```python
from build123d import *

# Parameters (mm, degrees)
EXTRUDE_1_DEPTH     = 165
SKETCH_2_W          = 10
SKETCH_2_H          = 150
CUT_EXTRUDE_1_DEPTH = 185.106287236
SKETCH_3_W          = 8
SKETCH_3_H          = 155
EXTRUDE_2_DEPTH     = 10
SKETCH_4_R          = 2.5
CUT_EXTRUDE_2_DEPTH = 180.638873855
SKETCH_5_W          = 20
SKETCH_5_H          = 3
EXTRUDE_3_DEPTH     = 10
CUT_EXTRUDE_3_DEPTH = 184.098675582


with BuildPart() as part:
    # 草圖1 → 填料-伸長1 (new body)
    with BuildSketch(Plane.XY):
        with BuildLine():
            Line((-57.75, 0), (-57.75, -10))
            Line((-57.75, -10), (-51.75, -10))
            Line((-51.75, -10), (-51.75, 0))
            ThreePointArc((-51.75, 0), (-1, 50.75), (49.75, 0))
            Line((49.75, 0), (57.75, 0))
            ThreePointArc((57.75, 0), (0, 57.75), (-57.75, 0))
        make_face()
    extrude(amount=EXTRUDE_1_DEPTH)

    # 草圖2 → 除料-伸長1 (cut, through all)
    with BuildSketch(Plane(origin=(0, 0, 0), x_dir=(1, 0, 0), z_dir=(0, 1, 0))):
        with Locations((-42.75, -80)):
            Rectangle(SKETCH_2_W, SKETCH_2_H)
        with Locations((-22.75, -80)):
            Rectangle(SKETCH_2_W, SKETCH_2_H)
        with Locations((-2.75, -80)):
            Rectangle(SKETCH_2_W, SKETCH_2_H)
        with Locations((17.25, -80)):
            Rectangle(SKETCH_2_W, SKETCH_2_H)
        with Locations((37.25, -80)):
            Rectangle(SKETCH_2_W, SKETCH_2_H)
    extrude(amount=CUT_EXTRUDE_1_DEPTH, mode=Mode.SUBTRACT)

    # 草圖3 → 填料-伸長2 (add)
    with BuildSketch(Plane.XZ):
        with Locations((53.75, 82.5)):
            Rectangle(SKETCH_3_W, SKETCH_3_H)
    extrude(amount=EXTRUDE_2_DEPTH)

    # 草圖4 → 除料-伸長2 (cut, through all)
    with BuildSketch(Plane.XY.offset(160)):
        with Locations((53.75, -5)):
            Circle(SKETCH_4_R)
    extrude(amount=-CUT_EXTRUDE_2_DEPTH, mode=Mode.SUBTRACT)

    # 草圖5 → 填料-伸長3 (add)
    with BuildSketch(Plane.ZY.offset(57.75)):
        with Locations((82.5, -8.5)):
            Rectangle(SKETCH_5_W, SKETCH_5_H)
    extrude(amount=EXTRUDE_3_DEPTH)

    # 草圖6 → 除料-伸長3 (cut, through all)
    with BuildSketch(Plane.XY.offset(160)):
        Polygon((57.75, -10), (57.75, -6), (51.75, -10), align=None)
    extrude(amount=-CUT_EXTRUDE_3_DEPTH, mode=Mode.SUBTRACT)


solid = part.part
```
Part model, mm, in its own coordinate system. A direction names the side the tool comes from. Round coordinates to 2 decimals unless told otherwise and drop trailing zeros. Loops run counter-clockwise (first coordinate to the right, second up) from the corner with the lowest first, then second, coordinate; pieces in that order, holes last. Notation, with made-up numbers: (19, 69) -> (58, 69) arc R18 cw to (58, 80) -> close; hole circle Ø4 at (19, 76.25). An arc over 180 degrees is marked (long way). Use CSV: the item, a comma, the result in double quotes. Start each with the question number.
1) Wall check: L1, parallel to Z at x = -6, y = 53; L2, parallel to X at y = 52.5, z = 56; L3, parallel to X at y = 38, z = 19. Give the ranges that are in metal, low to high. Write a range as [from, to].
2) Which spindle directions (+Z, -Z, +X, -X, +Y, -Y) get a long thin tool onto all of the face, cutting with end or side? Do faces 4 (the flat face through (-63, -7, 82)), 5 (the flat face through (-37.75, 39, 81)), 6 (the flat face through (37, 37, 155)), 7 (the flat face through (-51.75, -5, 81)). Say none if no direction does.
3) Drop flat-ended pins along their axis: P1, Ø10, axis at y = 36, z = 40, coming from the +X side; P2, Ø8, axis at x = 36, y = 32.5, coming from the -Z side; P3, Ø4, axis at y = 48, z = 74, coming from the +X side; P4, Ø6.5, axis at y = 26.5, z = 85, coming from the +X side. Give the stop position or say it passes through.
4) Pull direction Z, two halves, no side cores. Call faces 1 (the flat face through (0, 52, 165)), 2 (the flat face through (-7.75, 54, 81)), 3 (the flat face through (57.75, -3, 81)): +Z half, -Z half, draft (parallel to the pull), parting line (faces both ways), or undercut.
5) Cut at C-C, the plane x = 0. Write the cut outline in (y, z).
6) Cut at D-D, the plane y = 15.5. Write the cut outline in (x, z), plus the area to 3 significant figures.
7) Cut at A-A, the plane z = 60.5. Give the number of separate pieces and of enclosed holes in the cut face, plus the area to 3 significant figures.
Determined:
1,L1,"z = [0, 5], [155, 165]"
1,L2,"x = [-17.75, -7.75], [2.25, 12.25], [22.25, 24.06]"
1,L3,"x = [-37.75, -34.64], [42.25, 43.49]"
2,face 4,"+Z, -Z, -X, +Y"
2,face 5,"-X, +Y, -Y"
2,face 6,"+Y, -Y"
2,face 7,"+Z, -Z, -Y"
3,P1,"stops at x = 48.72"
3,P2,"stops at z = 0"
3,P3,"stops at x = 32.25"
3,P4,"stops at x = 52.86"
4,face 1,"+Z half"
4,face 2,"undercut"
4,face 3,"draft"
5,outline,"(50.74, 0) -> (57.75, 0) -> (57.75, 5) -> (50.74, 5) -> close; (50.74, 155) -> (57.75, 155) -> (57.75, 165) -> (50.74, 165) -> close"
6,outline,"(-55.63, 0) -> (-49.33, 0) -> (-49.33, 165) -> (-55.63, 165) -> close; (47.33, 0) -> (55.63, 0) -> (55.63, 165) -> (47.33, 165) -> close"
6,area,"2,410 mm2"
7,separate pieces,"6"
7,enclosed holes,"1"
7,area,"870 mm2"
